Source: three-view drawing plus pictorial views. Frame: mm from the lowest corner of the part. Round coordinates to 2 decimals unless told otherwise and drop trailing zeros. Order: outer loops, then holes, each group sorted by start corner. A loop starts at its lowest first (then second) coordinate and runs counter-clockwise, first axis right, second up. Notation, with made-up numbers: (-39, -28) -> (9, -28) arc R37 ccw to (9, 11) -> close; hole circle Ø9 at (66, 20). An arc over 180 degrees is marked (long way). Use a Markdown table: item, result.
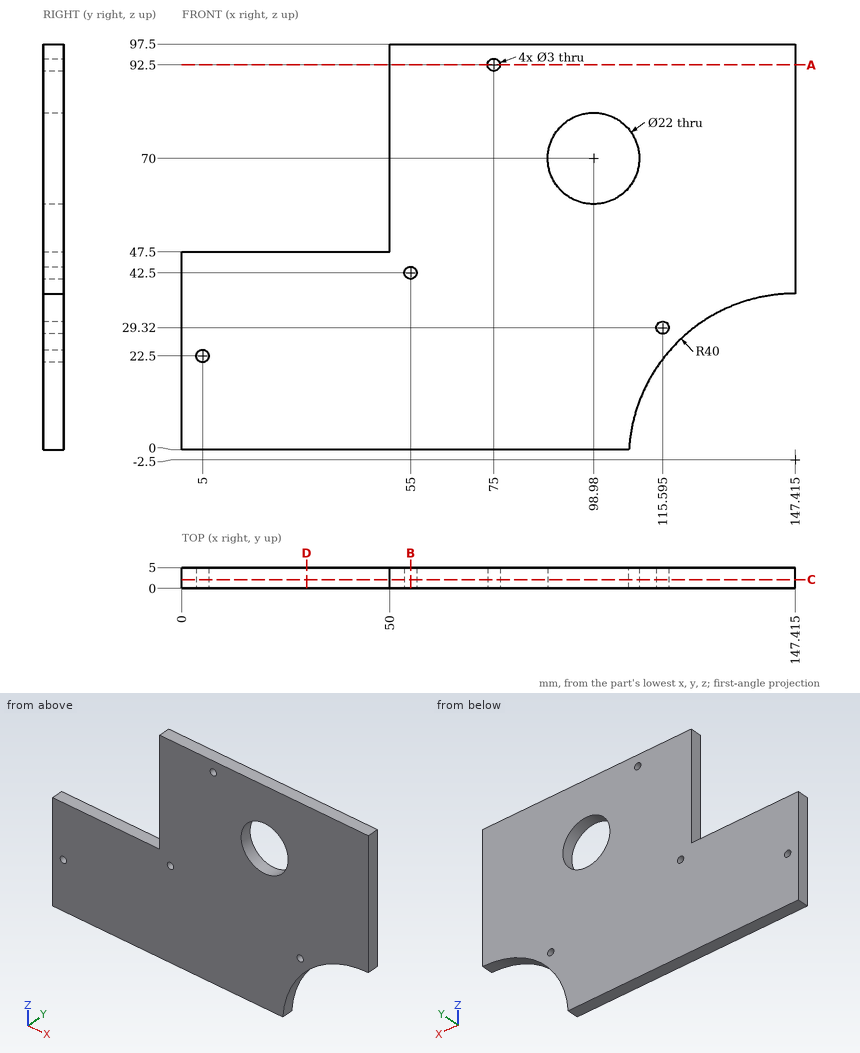
1) Cut plane B-B on x = 55. Return loops of the section in (y, z).
Results found:
| item | result |
|---|---|
| outline | (0, 0) -> (5, 0) -> (5, 41) -> (0, 41) -> close; (0, 44) -> (5, 44) -> (5, 97.5) -> (0, 97.5) -> close |
2) Line query: L1, parallel to X at y = 2, z = 70 (1 decimal); L2, parallel to Z at x = 75, y = 3; L3, parallel to Z at x = 5, y = 2.2. Output: solid intervals per line, ascending. Write a range as [from, to].
Results found:
| item | result |
|---|---|
| L1 | x = [50, 88], [110, 147.4] |
| L2 | z = [0, 91], [94, 97.5] |
| L3 | z = [0, 21], [24, 47.5] |
3) Cut plane C-C on y = 2.1. Return loops of the section in (x, z) (1 decimal).
Results found:
| item | result |
|---|---|
| outline | (0, 0) -> (107.5, 0) arc R40 cw to (147.4, 37.5) -> (147.4, 97.5) -> (50, 97.5) -> (50, 47.5) -> (0, 47.5) -> close; hole circle Ø3 at (5, 22.5); hole circle Ø3 at (55, 42.5); hole circle Ø3 at (75, 92.5); hole circle Ø22 at (99, 70); hole circle Ø3 at (115.6, 29.3) |
4) Pin query (flat end, axial travel): pin 1 Ø1.5 at (y, z) = (3, 73) entering from -X. Return the tip coordinate at first contact, or that it passes through.
Results found:
| item | result |
|---|---|
| pin 1 | stops at x = 50 |
5) Cut plane A-A on z = 92.5. Return loops of the section in (x, y) (1 decimal), and give its area (3 significant figures).
Results found:
| item | result |
|---|---|
| outline | (50, 0) -> (73.5, 0) -> (73.5, 5) -> (50, 5) -> close; (76.5, 0) -> (147.4, 0) -> (147.4, 5) -> (76.5, 5) -> close |
| area | 472 mm² |
6) Cut plane D-D on x = 30. Return loops of the section in (y, z).
Results found:
| item | result |
|---|---|
| outline | (0, 0) -> (5, 0) -> (5, 47.5) -> (0, 47.5) -> close |
